Part print with two shaded views. Sizes in mm from the minimum x, y, z corner. A direction names the side the tool comes from. Give positions to 0.01 mm unless a question says otherwise; leave off trailing zeros. Write each loop counter-clockwise with the first axis right and the second up, starting at its lowest first coordinate (ties: lowest second). Pieces come first, ordered by that corner, then holes. Notation, with made-up numbers: (43, 57) -> (52, 57) arc R11 cw to (52, 74) -> close; hole circle Ø3 at (36, 8). An arc over 180 degrees is marked (long way). Write item = value, one per line. Start each with the question number.
Q1. Saw through at A-A, the plane z = 3. List the corners of the cut face in (x, y).
Q2. Saw through at D-D, the plane z = 1.45. List the corners of the cut face in (x, y).
Q3. Drop flat-ended pins along their axis: P1, Ø1.6, axis at x = 6, z = 1.5, coming from the -Y side; P2, Ø0.5, axis at y = 0.5, z = 3.5, coming from the -X side; P3, Ø2.5, axis at x = 5.5, z = 3.5, coming from the +Y side. Give the stop position or say it passes through.
Q4. Tool access for the marked faces 1, 2 and 3: list every direction of +Z, -Z, +X, -X, +Y, -Y with a clear straight run to the whole face (end or side of a thin tool).
Q5. Saw through at C-C, the plane y = 0.4. List the corners of the cut face in (x, z).
Q6. Wall check: line 1 (Y direction, x = 6.5, z = 2.8); line 2 (X direction, y = 4.85, z = 1.35); line 3 (Z direction, x = 11, y = 5.55). Give the ranges that are in metal, low to high.
Q7. Saw through at B-B, the plane x = 14. List the corners of the cut face in (y, z), then the cut area to 3 significant figures.
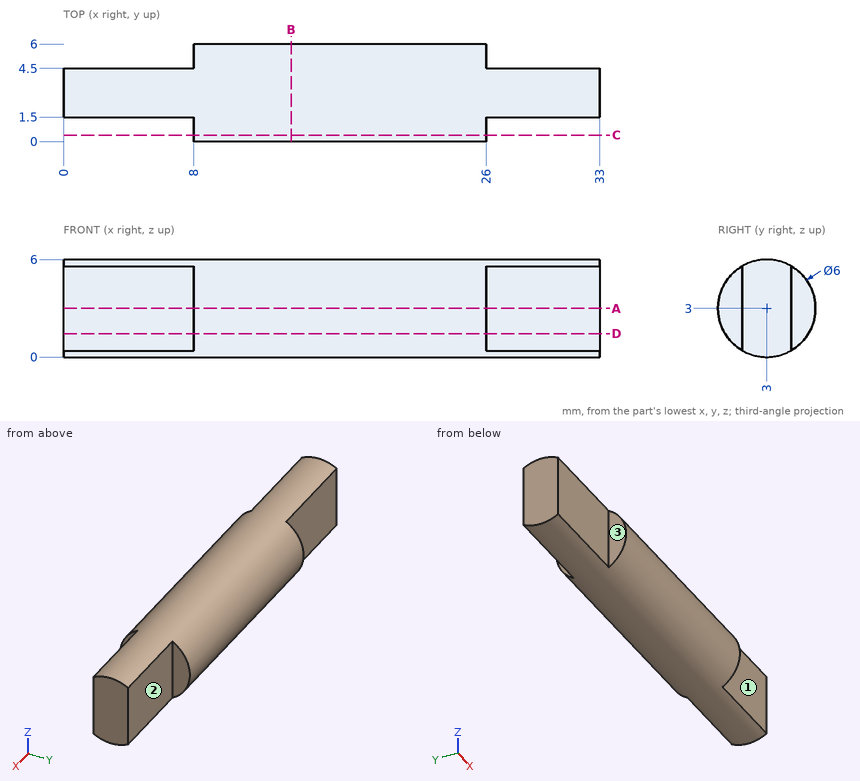
Report:
q1.outline = (0, 1.5) -> (8, 1.5) -> (8, 0) -> (26, 0) -> (26, 1.5) -> (33, 1.5) -> (33, 4.5) -> (26, 4.5) -> (26, 6) -> (8, 6) -> (8, 4.5) -> (0, 4.5) -> close
q2.outline = (0, 1.5) -> (8, 1.5) -> (8, 0.43) -> (26, 0.43) -> (26, 1.5) -> (33, 1.5) -> (33, 4.5) -> (26, 4.5) -> (26, 5.57) -> (8, 5.57) -> (8, 4.5) -> (0, 4.5) -> close
q3.P1 = 1.5
q3.P2 = 8
q3.P3 = 4.5
q4.face_1 = +Z, -Z, +X, -Y
q4.face_2 = +Z, -Z, +X, +Y
q4.face_3 = +Z, -Z, -X, -Y
q5.outline = (8, 1.5) -> (26, 1.5) -> (26, 4.5) -> (8, 4.5) -> close
q6.line_1 = 1.5 to 4.5
q6.line_2 = 8 to 26
q6.line_3 = 1.42 to 4.58
q7.outline = circle Ø6 at (3, 3)
q7.area = 28.3 mm2
